from build123d import *

# Parameters (mm, degrees)
SKETCH1_W           = 133.35
SKETCH1_H           = 37.465
BOSS_EXTRUDE1_DEPTH = 3.175
SKETCH2_W           = 126.492
SKETCH2_H           = 30.607
BOSS_EXTRUDE2_DEPTH = 0.79375
CUT_EXTRUDE1_DEPTH  = 3.96875
CUT_EXTRUDE2_REACH  = 5.969
SKETCH5_R           = 2
SKETCH6_R           = 3.175
CUT_EXTRUDE3_DEPTH  = 2


with BuildPart() as part:
    # Sketch1 → Boss-Extrude1 (new body)
    with BuildSketch(Plane(origin=(0, 0, 0), x_dir=(1, 0, 0), z_dir=(0, 1, 0))):
        Rectangle(SKETCH1_W, SKETCH1_H)
    extrude(amount=BOSS_EXTRUDE1_DEPTH)

    # Sketch2 → Boss-Extrude2 (add)
    with BuildSketch(Plane(origin=(0, 3.175, 0), x_dir=(1, 0, 0), z_dir=(0, 1, 0))):
        Rectangle(SKETCH2_W, SKETCH2_H)
    extrude(amount=BOSS_EXTRUDE2_DEPTH)

    # Sketch3 → Cut-Extrude1 (cut)
    with BuildSketch(Plane(origin=(0, 0, 0), x_dir=(1, 0, 0), z_dir=(0, 1, 0))):
        with BuildLine():
            Line((-9.525, -3.96875), (-58.7375, -3.96875))
            ThreePointArc((-58.7375, -3.96875), (-62.70625, 0), (-58.7375, 3.96875))
            Line((-58.7375, 3.96875), (-9.525, 3.96875))
            ThreePointArc((-9.525, 3.96875), (-5.55625, 0), (-9.525, -3.96875))
        make_face()
    cut_extrude1 = extrude(amount=CUT_EXTRUDE1_DEPTH, mode=Mode.SUBTRACT)

    # Mirror1: Cut-Extrude1 across plane
    add(cut_extrude1.mirror(Plane(origin=(0, 0, 0), x_dir=(0, 0, 1), z_dir=(1, 0, 0))), mode=Mode.SUBTRACT)

    # Sketch5 → Cut-Extrude2 (cut, up to next)
    with BuildSketch(Plane(origin=(0, 0, 0), x_dir=(1, 0, 0), z_dir=(0, 1, 0)), mode=Mode.PRIVATE) as cut_extrude2_sk1:
        with Locations((-57.15, -9.2075)):
            Circle(SKETCH5_R)
    cut_extrude2_tool1 = extrude(cut_extrude2_sk1.sketch, amount=CUT_EXTRUDE2_REACH, mode=Mode.PRIVATE) & part.part
    add(cut_extrude2_tool1.solids().sort_by_distance((-57.15, 0, 9.2075))[0], mode=Mode.SUBTRACT)
    # Sketch5 → Cut-Extrude2 (cut, up to next)
    with BuildSketch(Plane(origin=(0, 0, 0), x_dir=(1, 0, 0), z_dir=(0, 1, 0)), mode=Mode.PRIVATE) as cut_extrude2_sk2:
        with Locations((57.15, 9.2075)):
            Circle(SKETCH5_R)
    cut_extrude2_tool2 = extrude(cut_extrude2_sk2.sketch, amount=CUT_EXTRUDE2_REACH, mode=Mode.PRIVATE) & part.part
    add(cut_extrude2_tool2.solids().sort_by_distance((57.15, 0, -9.2075))[0], mode=Mode.SUBTRACT)

    # Sketch6 → Cut-Extrude3 (cut)
    with BuildSketch(Plane(origin=(0, 0, 0), x_dir=(-1, 0, 0), z_dir=(0, -1, 0))):
        with Locations((57.15, -9.2075)):
            Circle(SKETCH6_R)
        with Locations((-57.15, 9.2075)):
            Circle(SKETCH6_R)
    extrude(amount=-CUT_EXTRUDE3_DEPTH, mode=Mode.SUBTRACT)


solid = part.part
Work out the finished part from the listing and answer in its coordinate system (mm). A direction names the side the tool comes from. Round coordinates to 2 decimals unless told otherwise and drop trailing zeros. Loops run counter-clockwise (first coordinate to the right, second up) from the corner with the lowest first, then second, coordinate; pieces in that order, holes last. Notation, with made-up numbers: M 88,-9.75 L 97,-9.75 A13 cw 97,5.25 Z; hole C 52.25,80.5 d2. An arc over 180 degrees is marked long. One line per question, with ' | ' between items. Start each with the question number.
(1) A tool of negligible diameter and unlimited length cuts with its end or side. For faces 5 (the face through (-34, 2, 3.969)), 6 (the face through (-1, 2, 18.732)), 7 (the face through (-57.8, 2, 11.3)), from which of +Z, -Z, +X, -X, +Y, -Y can it reach the whole face along a straight path? Write none if from no direction.
(2) A cutting plane is placed at D-D on y = 1. Give the number of separate pieces and of enclosed holes in the cut face, plus the area to 3 significant figures.
(3) A flat-ended cylindrical pin translates along its axis: pin 1 Ø1.9 at (x, z) = (58.5, -10) entering from -Y. Find the tip coordinate at first contact, or state that the pin passes through.
(4) Find the intervals of material crossed by line 1 (Z direction, x = 57.15, y = 3.3); line 2 (Z direction, x = 57.15, y = 1.5); line 3 (Z direction, x = 32, y = 3.4), in increasing order.
(5) A cutting plane is placed at C-C on z = 0. Write down the section's boundary in (x, y) (3 decimals).
(6) A cutting plane is placed at A-A on x = 44. Write down the section's boundary in (y, z) (1 decimal), plus the area to 3 significant figures.
(7) A cutting plane is placed at B-B on x = -57.15. Write down the section's boundary in (y, z) (1 decimal).
(8) For a pull along X with two mould halves and no side action, classify faces 1 (the face through (-66.675, 2, 0)), 2 (the face through (34, 2, -3.969)), 3 (the face through (-53.978, 0.986, 9.068)), 4 (the face through (-1, 0, 0)) as released by +X, released by -X, zero draft, split by the parting line, or undercut.
Geometry check:
1) face 5: +Y, -Y | face 6: +Z, +X, -X, +Y, -Y | face 7: -Y
2) separate pieces: 1 | enclosed holes: 4 | area: 4,050 mm²
3) pin 1: stops at y = 2
4) line 1: z = -15.3 to -11.21, -7.21 to -3.97, 3.97 to 15.3 | line 2: z = -18.73 to -12.38, -6.03 to -3.97, 3.97 to 18.73 | line 3: z = -15.3 to -3.97, 3.97 to 15.3
5) outline: M -66.675,0 L -62.706,0 L -62.706,3.969 L -63.246,3.969 L -63.246,3.175 L -66.675,3.175 Z; M -5.556,0 L 5.556,0 L 5.556,3.969 L -5.556,3.969 Z; M 62.706,0 L 66.675,0 L 66.675,3.175 L 63.246,3.175 L 63.246,3.969 L 62.706,3.969 Z
6) outline: M 0,-18.7 L 3.2,-18.7 L 3.2,-15.3 L 4,-15.3 L 4,-4 L 0,-4 Z; M 0,4 L 4,4 L 4,15.3 L 3.2,15.3 L 3.2,18.7 L 0,18.7 Z | area: 112 mm²
7) outline: M 0,-18.7 L 3.2,-18.7 L 3.2,-15.3 L 4,-15.3 L 4,-4 L 0,-4 Z; M 0,4 L 4,4 L 4,7.2 L 2,7.2 L 2,6 L 0,6 Z; M 0,12.4 L 2,12.4 L 2,11.2 L 4,11.2 L 4,15.3 L 3.2,15.3 L 3.2,18.7 L 0,18.7 Z
8) face 1: released by -X | face 2: undercut | face 3: undercut | face 4: zero draft
